The model under review builds one solid part; all positions refer to its coordinate system, in mm. Face numbers are marked on the shaded views. A direction names the side the tool comes from. Coordinates: 2 decimals unless noted, no trailing zeros. Loops run counter-clockwise (first coordinate to the right, second up) from the corner with the lowest first, then second, coordinate; pieces in that order, holes last. Notation, with made-up numbers: (-24.75, 55.5) - (1.25, 55.5) arc R16 ccw to (1.25, 71.5) - close; hole circle Ø6 at (25.5, -15). An arc over 180 degrees is marked (long way). One line per item, written item: value. Start each with the question number.
1. To check wall thickness, follow line 1 (X direction, y = 1, z = 2.25); line 2 (X direction, y = -1.75, z = 2.8); line 3 (X direction, y = -0.5, z = 0.95). State the ranges of each line that lie inside material, in increasing order.
2. Insertion check: P1, Ø1, axis at x = -6.5, z = 0.5, coming from the -Y side; P2, Ø1, axis at x = 3.5, z = 0.5, coming from the +Y side; P3, Ø1, axis at y = -1, z = 2.5, coming from the -X side; P4, Ø2.5, axis at x = -7.5, y = 2.79, coming from the -Z side. Each pin has a flat end and moves straight along its axis. Give the tip position at first contact, or say it passes through.
3. For the marked faces 5 and 6, list the 3-axis set-ups (+Z, -Z, +X, -X, +Y, -Y) from which the entire face can be reached by the end or side of a thin tool; tool diameter is ignored.
4. We need section C-C, the plane x = 7.5. Give the boundary of the cut face in (y, z), then the cut area to 3 significant figures.
5. We need section B-B, the plane x = 0. Give the boundary of the cut face in (y, z), then the cut area to 3 significant figures.
6. Mouldability with a two-part tool opening along X and no side actions: class the marked faces 1, 2, 3 and 4 as +X half, -X half, draft (parallel to the pull), parting line (faces both ways), or undercut.
7. We need section D-D, the plane z = 1. Give the boundary of the cut face in (x, y), then the cut area to 3 significant figures.
8. We need section A-A, the plane y = 0. Give the boundary of the cut face in (x, z).
from build123d import *

# Parameters (mm, degrees)
SKETCH1_R           = 12.5
BOSS_EXTRUDE1_DEPTH = 3
CUT_EXTRUDE1_DEPTH  = 3
SKETCH3_R           = 2
CUT_EXTRUDE2_DEPTH  = 3


with BuildPart() as part:
    # Sketch1 → Boss-Extrude1 (new body)
    with BuildSketch(Plane.XY):
        Circle(SKETCH1_R)
    extrude(amount=BOSS_EXTRUDE1_DEPTH)

    # Sketch2 → Cut-Extrude1 (cut)
    with BuildSketch(Plane.XY.offset(3)):
        with BuildLine():
            Line((-1.249238699, 2.027252879), (2.006668261, 1.282042922))
            ThreePointArc((2.006668261, 1.282042922), (-0.531280863, -2.321226445), (-1.249238699, 2.027252879))
        make_face()
    extrude(amount=-CUT_EXTRUDE1_DEPTH, mode=Mode.SUBTRACT)

    # Sketch3 → Cut-Extrude2 (cut)
    with BuildSketch(Plane.XY.offset(3)):
        with Locations((-7.499150429, 2.786169925)):
            Circle(SKETCH3_R)
    extrude(amount=-CUT_EXTRUDE2_DEPTH, mode=Mode.SUBTRACT)


solid = part.part
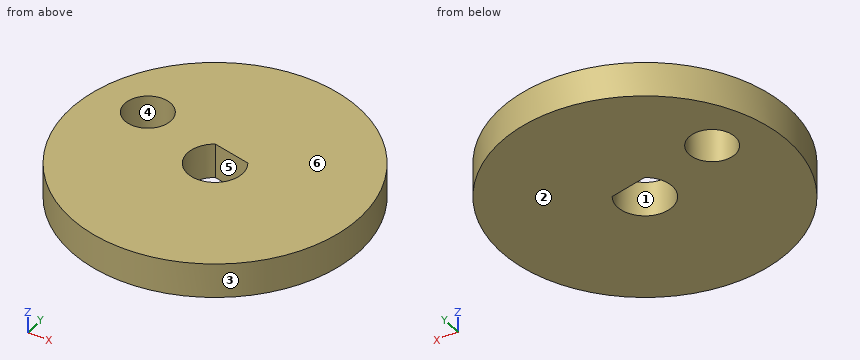
Findings below:
1. line 1: -12.46 to -8.4, -6.6 to -2.16, 2.16 to 12.46
1. line 2: -12.38 to -1.61, 1.61 to 12.38
1. line 3: -12.49 to -2.33, 2.33 to 12.49
2. P1: y = -10.97
2. P2: y = 12.13
2. P3: x = -12.49
2. P4: through
3. face 5: +Z, -Z
3. face 6: +Z, +X, -X, +Y, -Y
4. outline: (-10, 0) - (10, 0) - (10, 3) - (-10, 3) - close
4. area: 60.0 mm2
5. outline: (-12.5, 0) - (-2.38, 0) - (-2.38, 3) - (-12.5, 3) - close; (1.74, 0) - (12.5, 0) - (12.5, 3) - (1.74, 3) - close
5. area: 62.6 mm2
6. face 1: undercut
6. face 2: draft
6. face 3: parting line
6. face 4: undercut
7. outline: circle Ø25 at (0, 0); hole circle Ø4 at (-7.5, 2.79); hole (-1.25, 2.03) arc R2.38 ccw (long way) to (2.01, 1.28) - close
7. area: 462 mm2
8. outline: (-12.5, 0) - (-2.38, 0) - (-2.38, 3) - (-12.5, 3) - close; (2.38, 0) - (12.5, 0) - (12.5, 3) - (2.38, 3) - close
